The drawing under review shows one solid part. Ordinate dimensions are in mm from its lowest x, y, z. A direction names the side the tool comes from. Round coordinates to 2 decimals unless told otherwise and drop trailing zeros. Order: outer loops, then holes, each group sorted by start corner. A loop starts at its lowest first (then second) coordinate and runs counter-clockwise, first axis right, second up. Notation, with made-up numbers: M 36,16 L 49,16 A6 ccw 49,20 Z; hole C 87,-36 d2. An arc over 180 degrees is marked long. Answer as a JSON object with one key per item and string values. Group by question number.
1) For the marked faces 4, 5 and 6, list the 3-axis set-ups (+Z, -Z, +X, -X, +Y, -Y) from which the entire face can be reached by the end or side of a thin tool; tool diameter is ignored.
2) To check wall thickness, follow line 1 (Z direction, x = 4.6, y = 6.75); line 2 (Y direction, x = 4.5, z = 2.25) (1 decimal). State the ranges of each line that lie inside material, in increasing order.
3) The part is to be moulded in two halves that separate along Y. For the marked faces 1, 2 and 3, say which applies: +Y half, -Y half, draft (parallel to the pull), parting line (faces both ways), or undercut.
4) Consider section B-B, the plane y = 19.25. Write out the cut boundary in (x, z) (3 decimals).
5) Insertion check: pin 1 Ø1.5 at (x, y) = (5.5, 14.5) entering from -Z (3 decimals); pin 2 Ø1.6 at (y, z) = (17, 5) entering from -X; pin 3 Ø2 at (y, z) = (13, 5) entering from +X. Each pin has a flat end and moves straight along its axis. Give the tip position at first contact, or say it passes through.
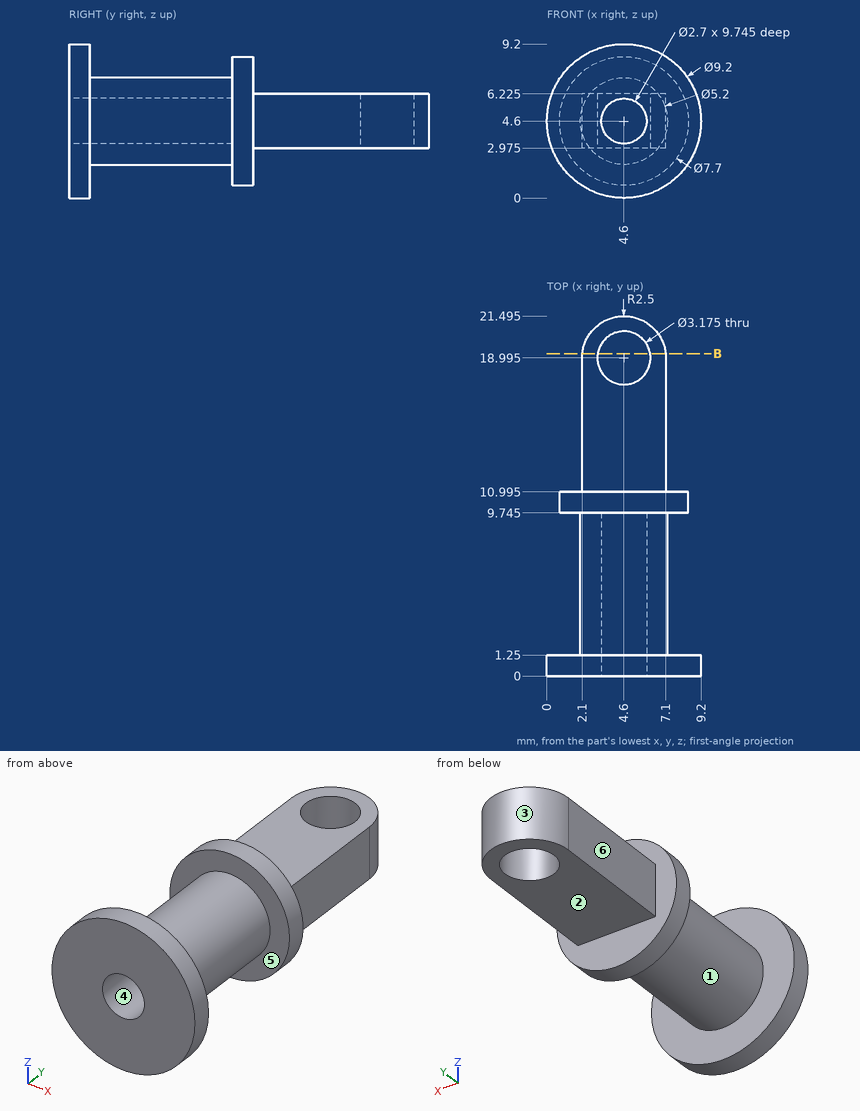
Results list:
{
 "1": {"face 4": "-Y", "face 5": "none", "face 6": "+Z, -Z, -X, +Y"},
 "2": {"line 1": "2 to 3.25, 5.95 to 7.2", "line 2": "0 to 11"},
 "3": {"face 1": "undercut", "face 2": "draft", "face 3": "+Y half"},
 "4": {"outline": "M 2.113,2.975 L 3.033,2.975 L 3.033,6.225 L 2.113,6.225 Z; M 6.167,2.975 L 7.087,2.975 L 7.087,6.225 L 6.167,6.225 Z"},
 "5": {"pin 1": "z = 2.975", "pin 2": "x = 2.1", "pin 3": "x = 7.1"}
}
